For this review, take the finished solid that the model builds, in its own axes (mm). Coordinates: 2 decimals unless noted, no trailing zeros. Order: outer loops, then holes, each group sorted by start corner. A loop starts at its lowest first (then second) coordinate and runs counter-clockwise, first axis right, second up. Notation, with made-up numbers: (57.5, -29.5) -> (102.5, -29.5) arc R10 ccw to (102.5, -18.5) -> close; hole circle Ø5 at (-38, -22). An arc over 180 degrees is marked (long way). Write item = value, one per line. Start each with the question number.
1) Consider section C-C on y = 20. Give the boundary of the cut face in (x, z).
2) Consider section B-B on x = 1.8. Give the boundary of the cut face in (y, z).
3) Consider section A-A on z = 0. Give the boundary of the cut face in (x, y), and give its area (3 significant figures).
4) Wall thickness on probe 1 along X at (y, z) = (25.5, -21); probe 2 along Z at (x, y) = (2.3, -19.5); probe 3 along Z at (x, y) = (1.35, 15): over which ranges is each line inside the solid? List them lowest first. Write a range as [from, to].
5) Insertion check: pin 1 Ø1.1 at (x, y) = (3.5, -0.5) entering from -Z; pin 2 Ø0.5 at (x, y) = (3.5, -0.5) entering from -Z; pin 3 Ø1.5 at (x, z) = (2, -21) entering from +Y. Each pin has a flat end and moves straight along its axis. Give the tip position at first contact, or say it passes through.
from build123d import *

# Parameters (mm, degrees)
CROQUIS1_R              = 37.5
SALIENTE_EXTRUIR1_DEPTH = 3
CROQUIS3_W              = 2.216229218
CROQUIS3_H              = 1.031247755
CROQUIS3_W_2            = 2.277685896
SALIENTE_EXTRUIR2_DEPTH = 1
CORTAR_EXTRUIR1_DEPTH   = 20
CROQUIS5_R              = 0.35967939
CROQUIS5_R_2            = 0.365171254
CROQUIS5_R_3            = 0.400306504
CORTAR_EXTRUIR2_DEPTH   = 20


with BuildPart() as part:
    # Croquis1 → Saliente-Extruir1 (new body)
    with BuildSketch(Plane(origin=(0, 0, 0), x_dir=(0, 0, -1), z_dir=(1, 0, 0))):
        Circle(CROQUIS1_R)
    extrude(amount=SALIENTE_EXTRUIR1_DEPTH)

    # Croquis3 → Saliente-Extruir2 (add)
    with BuildSketch(Plane(origin=(3, 0, 0), x_dir=(0, 0, -1), z_dir=(1, 0, 0))):
        with Locations((16.1, -0.515623878)):
            Rectangle(CROQUIS3_W, CROQUIS3_H)
        with Locations((23.8, -0.515623878)):
            Rectangle(CROQUIS3_W_2, CROQUIS3_H)
        with Locations((31.2, -0.515623878)):
            Rectangle(CROQUIS3_W_2, CROQUIS3_H)
    extrude(amount=SALIENTE_EXTRUIR2_DEPTH)

    # Croquis4 → Cortar-Extruir1 (cut)
    with BuildSketch(Plane(origin=(0, 0, -32.338842948), x_dir=(-1, 0, 0), z_dir=(0, 0, -1))):
        with BuildLine():
            add(Edge.make_bspline(
                [(-3, 0), (-4, -0.257811939), (-4, -0.515623877)],
                knots=[0, 0, 0, 0.5, 0.5, 0.5], degree=2))
            Line((-3, 0), (-4, 0))
            Line((-4, 0), (-4, -0.515623877))
        make_face()
        with BuildLine():
            Line((-4, -1.031247755), (-3, -1.031247755))
            add(Edge.make_bspline(
                [(-4, -0.515623877), (-4, -0.773435816), (-3, -1.031247755)],
                knots=[0.5, 0.5, 0.5, 1, 1, 1], degree=2))
            Line((-4, -0.515623877), (-4, -1.031247755))
        make_face()
    extrude(amount=-CORTAR_EXTRUIR1_DEPTH, mode=Mode.SUBTRACT)

    # Croquis5 → Cortar-Extruir2 (cut)
    with BuildSketch(Plane(origin=(3, 0, 0), x_dir=(0, 0, -1), z_dir=(1, 0, 0))):
        with Locations((17.58621928, -0.515623877)):
            Circle(CROQUIS5_R)
        with Locations((25.380798287, -0.515623877)):
            Circle(CROQUIS5_R_2)
        with Locations((32.915617677, -0.515623877)):
            Circle(CROQUIS5_R_3)
    extrude(amount=-CORTAR_EXTRUIR2_DEPTH, mode=Mode.SUBTRACT)


solid = part.part
Answer sheet:
q1.outline = (0, -31.72) -> (3, -31.72) -> (3, 31.72) -> (0, 31.72) -> close
q2.outline = circle Ø75 at (0, 0); hole circle Ø0.8 at (-0.52, -32.92); hole circle Ø0.73 at (-0.52, -25.38); hole circle Ø0.72 at (-0.52, -17.59)
q3.outline = (0, -37.5) -> (3, -37.5) -> (3, 37.5) -> (0, 37.5) -> close
q3.area = 225 mm2
q4.probe_1 = [0, 3]
q4.probe_2 = [-32.03, 32.03]
q4.probe_3 = [-34.37, 34.37]
q5.pin_1 = -37.5
q5.pin_2 = -32.34
q5.pin_3 = 31.56
